from build123d import *

# Parameters (mm, degrees)
BOSS_EXTRUDE1_DEPTH = 10
SKETCH2_R           = 1.25
BOSS_EXTRUDE2_DEPTH = 8
SKETCH3_R           = 1.25
CUT_EXTRUDE1_DEPTH  = 8


with BuildPart() as part:
    # Sketch1 → Boss-Extrude1 (new body)
    with BuildSketch(Plane(origin=(0, 0, 0), x_dir=(1, 0, 0), z_dir=(0, 1, 0))):
        Polygon((0, 2.886751346), (-2.5, 1.443375673), (-2.5, -1.443375673), (0, -2.886751346), (2.5, -1.443375673), (2.5, 1.443375673), align=None)
    extrude(amount=BOSS_EXTRUDE1_DEPTH)

    # Sketch2 → Boss-Extrude2 (add)
    with BuildSketch(Plane(origin=(0, 10, 0), x_dir=(1, 0, 0), z_dir=(0, 1, 0))):
        Circle(SKETCH2_R)
    extrude(amount=BOSS_EXTRUDE2_DEPTH)

    # Sketch3 → Cut-Extrude1 (cut)
    with BuildSketch(Plane(origin=(0, 0, 0), x_dir=(-1, 0, 0), z_dir=(0, -1, 0))):
        Circle(SKETCH3_R)
    extrude(amount=-CUT_EXTRUDE1_DEPTH, mode=Mode.SUBTRACT)


solid = part.part
Could you check a few things on this model? Use its own coordinates, in mm. A direction names the side the tool comes from. Round coordinates to 2 decimals unless told otherwise and drop trailing zeros. Order: outer loops, then holes, each group sorted by start corner. A loop starts at its lowest first (then second) coordinate and runs counter-clockwise, first axis right, second up.
(1) Imagine slicing it at B-B (z = 0). Write out the boundary of the cut face in (x, y), plus the area to 3 significant figures.
Response values:
outline: (-2.5, 0) - (-1.25, 0) - (-1.25, 8) - (1.25, 8) - (1.25, 0) - (2.5, 0) - (2.5, 10) - (1.25, 10) - (1.25, 18) - (-1.25, 18) - (-1.25, 10) - (-2.5, 10) - close
area: 50.0 mm2
(2) If we mould it in two halves opening along Z, with no side actions, what happens to faces 4 (the flat face through (-1, 0, 1)), 5 (the cylindrical face through (0.27, 3.94, 1.22)), 6 (the flat face through (1.233, 4.93, 2.175))? For each: released by +Z, released by -Z, zero draft, split by the parting line, or undercut.
Response values:
face 4: zero draft
face 5: undercut
face 6: released by +Z
(3) Imagine slicing it at A-A (y = 1). Write out the boundary of the cut face in (x, z).
Response values:
outline: (-2.5, -1.44) - (0, -2.89) - (2.5, -1.44) - (2.5, 1.44) - (0, 2.89) - (-2.5, 1.44) - close; hole circle Ø2.5 at (0, 0)
(4) Which directions (+Z, -Z, +X, -X, +Y, -Y) give clear straight access to the entire face, cutting with the end or side of a thin tool? Please do faces 1 (the cylindrical face through (-0.27, 13.94, 1.22)), 2 (the flat face through (0, 8, 0)), 3 (the flat face through (-1.267, 4.93, 2.155)).
Response values:
face 1: +Y
face 2: -Y
face 3: +Z, -X, +Y, -Y
(5) I'm going to push a flat-ended pin straight in: pin 1 (1.5 mm diameter, centred on x = 0.5, y = 15.5, fed in from +Z). Where does the tip first touch, or does it pass through?
Response values:
pin 1: stops at z = 1.25
(6) Imagine slicing it at C-C (y = 9.5). Write out the boundary of the cut face in (x, z), plus the area to 3 significant figures.
Response values:
outline: (-2.5, -1.44) - (0, -2.89) - (2.5, -1.44) - (2.5, 1.44) - (0, 2.89) - (-2.5, 1.44) - close
area: 21.7 mm2
(7) Imagine slicing it at D-D (x = -0.4). Write out the boundary of the cut face in (y, z).
Response values:
outline: (0, -2.66) - (10, -2.66) - (10, -1.18) - (18, -1.18) - (18, 1.18) - (10, 1.18) - (10, 2.66) - (0, 2.66) - (0, 1.18) - (8, 1.18) - (8, -1.18) - (0, -1.18) - close
(8) Please list where these lines run through material, in increasing order: line 1 along X through (y, z) = (4.75, 0); line 2 along X through (y, z) = (4, -0.9); line 3 along Y through (x, z) = (1.35, -1.65).
Response values:
line 1: x = -2.5 to -1.25, 1.25 to 2.5
line 2: x = -2.5 to -0.87, 0.87 to 2.5
line 3: y = 0 to 10
